```python
from build123d import *

# Parameters (mm, degrees)
BOSS_EXTRUDE2_DEPTH = 2.5
SKETCH5_R           = 3.75
CUT_EXTRUDE2_DEPTH  = 5
CUT_EXTRUDE3_DEPTH  = 10


with BuildPart() as part:
    # Sketch3 → Boss-Extrude2 (new, symmetric)
    with BuildSketch(Plane(origin=(0, 0, 0), x_dir=(1, 0, 0), z_dir=(0, 1, 0))):
        with BuildLine():
            Line((70, 30), (70, 10))
            ThreePointArc((70, 10), (67.071067812, 2.928932188), (60, 0))
            Line((60, 0), (-60, 0))
            ThreePointArc((-60, 0), (-67.071067812, 2.928932188), (-70, 10))
            Line((-70, 10), (-70, 30))
            ThreePointArc((-70, 30), (-68.535533906, 33.535533906), (-65, 35))
            Line((-65, 35), (-45, 35))
            Line((-45, 35), (-45, 103))
            Line((-45, 103), (-60, 103))
            ThreePointArc((-60, 103), (-67.071067812, 105.928932188), (-70, 113))
            Line((-70, 113), (-70, 147))
            ThreePointArc((-70, 147), (-67.071067812, 154.071067812), (-60, 157))
            Line((-60, 157), (-45, 157))
            Line((-45, 157), (-45, 225))
            Line((-45, 225), (-65.064414928, 225))
            ThreePointArc((-65.064414928, 225), (-68.304785278, 226.192113447), (-70, 229.2))
            Line((-70, 229.2), (-70, 245))
            ThreePointArc((-70, 245), (-66.467868189, 254.855318839), (-57.35, 260))
            Line((-57.35, 260), (57.35, 260))
            ThreePointArc((57.35, 260), (66.467868189, 254.855318839), (70, 245))
            Line((70, 245), (70, 229.2))
            ThreePointArc((70, 229.2), (68.304785278, 226.192113447), (65.064414928, 225))
            Line((65.064414928, 225), (45, 225))
            Line((45, 225), (45, 157))
            Line((45, 157), (60, 157))
            ThreePointArc((60, 157), (67.071067812, 154.071067812), (70, 147))
            Line((70, 147), (70, 113))
            ThreePointArc((70, 113), (67.071067812, 105.928932188), (60, 103))
            Line((60, 103), (45, 103))
            Line((45, 103), (45, 35))
            Line((45, 35), (65, 35))
            ThreePointArc((65, 35), (68.535533906, 33.535533906), (70, 30))
        make_face()
    extrude(amount=BOSS_EXTRUDE2_DEPTH, both=True)

    # Sketch5 → Cut-Extrude2 (cut)
    with BuildSketch(Plane(origin=(0, 2.5, 0), x_dir=(1, 0, 0), z_dir=(0, 1, 0))):
        with Locations(Location((-25, 75, 0), (0, 0, 270))):
            Circle(SKETCH5_R)
        with Locations(Location((-22.5, 202.5, 0), (0, 0, 270))):
            Circle(SKETCH5_R)
        with Locations(Location((-15, 185, 0), (0, 0, 270))):
            Circle(SKETCH5_R)
        with Locations(Location((25, 75, 0), (0, 0, 270))):
            Circle(SKETCH5_R)
        with Locations(Location((15, 185, 0), (0, 0, 270))):
            Circle(SKETCH5_R)
        with Locations(Location((22.5, 202.5, 0), (0, 0, 270))):
            Circle(SKETCH5_R)
    extrude(amount=-CUT_EXTRUDE2_DEPTH, mode=Mode.SUBTRACT)

    # Sketch6 → Cut-Extrude3 (cut)
    with BuildSketch(Plane(origin=(0, 2.5, 0), x_dir=(1, 0, 0), z_dir=(0, 1, 0))):
        with BuildLine():
            Line((-45, 157), (-45, 103))
            Line((-45, 103), (-60, 103))
            ThreePointArc((-60, 103), (-67.071067812, 105.928932188), (-70, 113))
            Line((-70, 113), (-70, 147))
            ThreePointArc((-70, 147), (-67.071067812, 154.071067812), (-60, 157))
            Line((-60, 157), (-45, 157))
        make_face()
        with BuildLine():
            Line((-45, 35), (45, 35))
            Line((45, 35), (65, 35))
            ThreePointArc((65, 35), (68.535533906, 33.535533906), (70, 30))
            Line((70, 30), (70, 10))
            ThreePointArc((70, 10), (67.071067812, 2.928932188), (60, 0))
            Line((60, 0), (-60, 0))
            ThreePointArc((-60, 0), (-67.071067812, 2.928932188), (-70, 10))
            Line((-70, 10), (-70, 30))
            ThreePointArc((-70, 30), (-68.535533906, 33.535533906), (-65, 35))
            Line((-65, 35), (-45, 35))
        make_face()
        with BuildLine():
            Line((45, 157), (45, 103))
            Line((45, 103), (60, 103))
            ThreePointArc((60, 103), (67.071067812, 105.928932188), (70, 113))
            Line((70, 113), (70, 147))
            ThreePointArc((70, 147), (67.071067812, 154.071067812), (60, 157))
            Line((60, 157), (45, 157))
        make_face()
        with BuildLine():
            Line((-45, 225), (45, 225))
            Line((45, 225), (65.064414928, 225))
            ThreePointArc((65.064414928, 225), (68.304785278, 226.192113447), (70, 229.2))
            Line((70, 229.2), (70, 245))
            ThreePointArc((70, 245), (66.467868189, 254.855318839), (57.35, 260))
            Line((57.35, 260), (-57.35, 260))
            ThreePointArc((-57.35, 260), (-66.467868189, 254.855318839), (-70, 245))
            Line((-70, 245), (-70, 229.2))
            ThreePointArc((-70, 229.2), (-68.304785278, 226.192113447), (-65.064414928, 225))
            Line((-65.064414928, 225), (-45, 225))
        make_face()
    extrude(amount=-CUT_EXTRUDE3_DEPTH, mode=Mode.SUBTRACT)


solid = part.part
```
Design review of the part built by this model. Coordinates are the model's own, in mm. Give positions to 0.01 mm unless a question says otherwise; leave off trailing zeros. Loops run counter-clockwise (first coordinate to the right, second up) from the corner with the lowest first, then second, coordinate; pieces in that order, holes last. Notation, with made-up numbers: (63, -4.5) -> (99, -4.5) arc R35 ccw to (99, 33.5) -> close; hole circle Ø1 at (52, 27.5). An arc over 180 degrees is marked (long way). Write each question's results on one line, items separated by ' | '.
Q1. Take a section at C-C, the plane x = 15. Write out the cut boundary in (y, z), plus the area to 4 significant figures.
Reply:
outline: (-2.5, -225) -> (2.5, -225) -> (2.5, -188.75) -> (-2.5, -188.75) -> close; (-2.5, -181.25) -> (2.5, -181.25) -> (2.5, -35) -> (-2.5, -35) -> close | area: 912.5 mm²
Q2. The part is to be moulded in two halves that separate along X. For faces 1 (the face through (-12.466, 0.035, -187.764)), 2 (the face through (1, -2.5, -131)), 3 (the face through (-45, 0, -129)), say which applies: +X half, -X half, draft (parallel to the pull), parting line (faces both ways), or undercut.
Reply:
face 1: undercut | face 2: draft | face 3: -X half
Q3. Take a section at B-B, the plane y = -1.7. Write out the cut boundary in (x, z), plus the area to 3 significant figures.
Reply:
outline: (-45, -225) -> (45, -225) -> (45, -35) -> (-45, -35) -> close; hole circle Ø7.5 at (-25, -75); hole circle Ø7.5 at (-22.5, -202.5); hole circle Ø7.5 at (-15, -185); hole circle Ø7.5 at (15, -185); hole circle Ø7.5 at (22.5, -202.5); hole circle Ø7.5 at (25, -75) | area: 16,800 mm²
Q4. For pin 1 Ø8.5 at (x, z) = (15, -185) entering from +Y; pin 2 Ø6 at (x, z) = (-15, -185) entering from -Y, all flat-tipped, find the tip position at first contact; note any pin that passes through.
Reply:
pin 1: stops at y = 2.5 | pin 2: passes through
Q5. Take a section at A-A, the plane z = -185. Write out the cut boundary in (x, y), plus the area to 3 significant figures.
Reply:
outline: (-45, -2.5) -> (-18.75, -2.5) -> (-18.75, 2.5) -> (-45, 2.5) -> close; (-11.25, -2.5) -> (11.25, -2.5) -> (11.25, 2.5) -> (-11.25, 2.5) -> close; (18.75, -2.5) -> (45, -2.5) -> (45, 2.5) -> (18.75, 2.5) -> close | area: 375 mm²
Q6. Wall thickness on L1, parallel to X at y = 0.15, z = -202.5; L2, parallel to X at y = 0.4, z = -75; L3, parallel to Z at x = 20.5, y = 0.4: over which ranges is each line inside the solid? List them lowest first.
Reply:
L1: x = -45 to -26.25, -18.75 to 18.75, 26.25 to 45 | L2: x = -45 to -28.75, -21.25 to 21.25, 28.75 to 45 | L3: z = -225 to -205.67, -199.33 to -35
